```python
from build123d import *

# Parameters (mm, degrees)
SKETCH1_W                = 1000
SKETCH1_H                = 1000
BOSS_EXTRUDE1_DEPTH      = 100
SKETCH2_W                = 1050
SKETCH2_H                = 1050
SKETCH2_W_2              = 1000
SKETCH2_H_2              = 1000
BOSS_EXTRUDE3_DEPTH      = 200
SKETCH3_W                = 25
SKETCH3_H                = 30
BOSS_EXTRUDE4_DEPTH      = 25
FILLET1_R                = 2.5
FILLET2_R                = 10
SKETCH5_R                = 5
BOSS_EXTRUDE5_DEPTH      = 32.5
BOSS_EXTRUDE5_DEPTH_BACK = 32.5


with BuildPart() as part:
    # Sketch1 → Boss-Extrude1 (new body)
    with BuildSketch(Plane(origin=(0, 0, 0), x_dir=(1, 0, 0), z_dir=(0, 1, 0))):
        Rectangle(SKETCH1_W, SKETCH1_H)
    extrude(amount=BOSS_EXTRUDE1_DEPTH)

    # Sketch2 → Boss-Extrude3 (add)
    with BuildSketch(Plane(origin=(0, 0, 0), x_dir=(1, 0, 0), z_dir=(0, 1, 0))):
        Rectangle(SKETCH2_W, SKETCH2_H)
        Rectangle(SKETCH2_W_2, SKETCH2_H_2, mode=Mode.SUBTRACT)
    extrude(amount=BOSS_EXTRUDE3_DEPTH)

    # Sketch3 → Boss-Extrude4 (add)
    with BuildSketch(Plane.XZ):
        Rectangle(SKETCH3_W, SKETCH3_H)
    extrude(amount=BOSS_EXTRUDE4_DEPTH)

    # Fillet1
    fillet1_edges = [part.edges().sort_by_distance(p)[0] for p in [
        (12.5, 0, 0),
        (0, 0, 15),
        (-12.5, 0, 0),
        (0, 0, -15),
    ]]
    fillet(fillet1_edges, radius=FILLET1_R)

    # Fillet2
    fillet2_edges = [part.edges().sort_by_distance(p)[0] for p in [
        (12.5, -25, 0),
        (-12.5, -25, 0),
    ]]
    fillet(fillet2_edges, radius=FILLET2_R)

    # Sketch5 → Boss-Extrude5 (add, two sides)
    with BuildSketch(Plane.XY) as boss_extrude5_sk:
        with Locations((0, -17.5)):
            Circle(SKETCH5_R)
    extrude(amount=BOSS_EXTRUDE5_DEPTH)
    extrude(boss_extrude5_sk.sketch, amount=-BOSS_EXTRUDE5_DEPTH_BACK)


solid = part.part
```
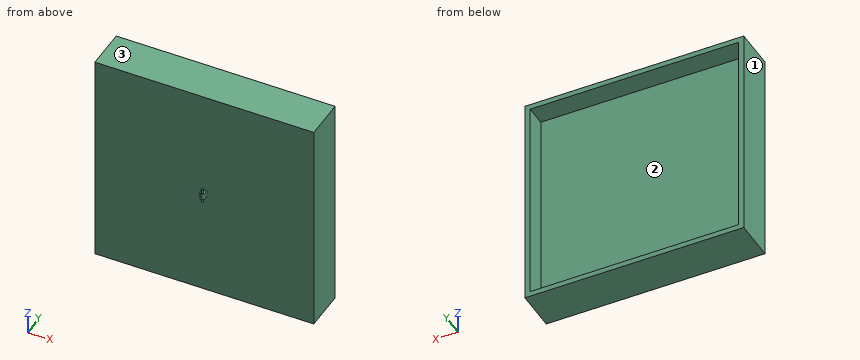
Geometry check sheet. Reference: the model listing, model coordinates, mm. Face numbers are marked on the shaded views. Give positions to 0.01 mm unless a question says otherwise; leave off trailing zeros. Loops run counter-clockwise (first coordinate to the right, second up) from the corner with the lowest first, then second, coordinate; pieces in that order, holes last. Notation, with made-up numbers: M -18.5,-16.75 L -9.5,-16.75 A27 cw -9.5,21.25 Z; hole C 5,47.25 d10. An arc over 180 degrees is marked long. Write item = value, one per line.
(1) Sectioned sample at A-A, the plane x = -113. Record the cut outline in (y, z), plus the area to 3 significant figures.
Answer below:
outline = M 0,-525 L 200,-525 L 200,-500 L 100,-500 L 100,500 L 200,500 L 200,525 L 0,525 Z
area = 110,000 mm2
(2) Sectioned sample at B-B, the plane z = 338.5. Record the cut outline in (x, y).
Answer below:
outline = M -525,0 L 525,0 L 525,200 L 500,200 L 500,100 L -500,100 L -500,200 L -525,200 Z
(3) Release check for a two-part mould opening along Z. For the marked faces 1, 2 and 3 record: released by +Z, released by -Z, zero draft, split by the parting line, or undercut.
Answer below:
face_1 = zero draft
face_2 = undercut
face_3 = released by +Z
(4) Gauge pin test, flat ends, axial feed: pin 1 Ø5 at (x, y) = (-0.5, -17) entering from -Z; pin 2 Ø4 at (y, z) = (-11.5, 0) entering from +X; pin 3 Ø3 at (x, y) = (2.5, -19.5) entering from +Z. Record the tip position at first contact, or that the pin passes through.
Answer below:
pin_1 = -32.5
pin_2 = 12.5
pin_3 = 32.5
(5) Material ranges on line 1 (Z direction, x = 439.5, y = 147); line 2 (Y direction, x = 239.5, z = -149), recorded low to high. Write a range as [from, to].
Answer below:
line_1 = [-525, -500], [500, 525]
line_2 = [0, 100]
